Autodesk Inventor part; units mm, degrees
ref_plane "YZ Plane" through (0, 0, 0) normal (1, 0, 0) x (0, 1, 0)
ref_plane "XZ Plane" through (0, 0, 0) normal (0, 1, 0) x (-1, 0, 0)
ref_plane "XY Plane" through (0, 0, 0) normal (0, 0, 1) x (1, 0, 0)
sketch "Sketch1" plane through (0, 0, 0) normal (0, 0, 1) x (1, 0, 0)
  line L0 (-266.7, 101.6) -> (-342.9, 101.6)
  line L1 (-342.9, 101.6) -> (-342.9, 0)
  line L2 (-342.9, 0) -> (342.9, 0)
  line L3 (342.9, 0) -> (342.9, 101.6)
  line L4 (342.9, 101.6) -> (266.7, 101.6)
  line L5 (266.7, 101.6) -> (266.7, 2.54)
  line L6 (266.7, 2.54) -> (-266.7, 2.54)
  line L7 (-266.7, 2.54) -> (-266.7, 101.6)
  point P0 (0, 0)
  point P1 (0, 0)
  point P2 (0, 2.54)
  dimension "d0" = 685.8
  dimension "d1" = 101.6
  dimension "d2" = 76.2
  dimension "d3" = 2.54
extrude "Extrusion1" add sketch "Sketch1" along normal mid plane 939.8
sketch "Sketch2" plane through (0, 0, -469.9) normal (0, 0, -1) x (-1, 0, 0)
  line L0 (-342.9, 0) -> (-342.9, 101.6)
  line L1 (342.9, 0) -> (-342.9, 0)
  line L2 (-342.9, 101.6) -> (342.9, 101.6)
  line L3 (342.9, 101.6) -> (342.9, 0)
  line L4 (342.9, 0) -> (-342.9, 0)
  line L5 (-342.9, 0) -> (-342.9, 101.6)
  point P0 (0, 0)
extrude "Extrusion2" add sketch "Sketch2" along normal blind 2.54
sketch "Sketch3" plane through (-266.7, 2.54, 469.9) normal (0, 1, 0) x (1, 0, 0)
  line L0 (0, 0) -> (533.4, 0)
  line L1 (533.4, 939.8) -> (533.4, 0)
  line L2 (0, 939.8) -> (0, 0)
  line L3 (0, 152.4) -> (533.4, 152.4)
  line L4 (533.4, 152.4) -> (533.4, 228.6)
  line L5 (533.4, 228.6) -> (0, 228.6)
  line L6 (0, 228.6) -> (0, 152.4)
  line L7 (0, 533.4) -> (152.4, 533.4)
  line L8 (152.4, 533.4) -> (152.4, 406.4)
  line L9 (152.4, 406.4) -> (0, 406.4)
  line L10 (0, 406.4) -> (0, 533.4)
  line L11 (381, 533.4) -> (533.4, 533.4)
  line L12 (533.4, 533.4) -> (533.4, 406.4)
  line L13 (533.4, 406.4) -> (381, 406.4)
  line L14 (381, 406.4) -> (381, 533.4)
  point P0 (266.7, 469.9)
  point P1 (152.4, 469.9)
  dimension "d8" = 76.2
  dimension "d9" = 152.4
  dimension "d31" = 152.4
  dimension "d32" = 127
extrude "Extrusion7" cut sketch "Sketch3" against normal up to next contours L2 L3 L1 L0
extrude "Extrusion3" add sketch "Sketch3" along normal blind 25.4 contours L2 L5 L1 L3
extrude "Extrusion8" add sketch "Sketch3" along normal blind 127 contours L2 L7 L8 L9 | L13 L14 L11 L1
sketch "Sketch4" plane through (-342.9, 0, 469.9) normal (0, -1, 0) x (1, 0, 0)
  line L0 (685.8, 0) -> (0, 0)
  line L1 (0, -942.34) -> (0, 0)
  line L2 (0, -942.34) -> (685.8, -942.34)
  line L3 (76.2, -939.8) -> (76.2, -228.6)
  line L4 (342.9, -469.9) -> (342.9, 0) construction
  line L5 (12.7, -929.64) -> (63.5, -929.64)
  line L6 (63.5, -929.64) -> (63.5, -12.7)
  line L7 (63.5, -12.7) -> (12.7, -12.7)
  line L8 (12.7, -12.7) -> (12.7, -929.64)
  line L9 (673.1, -929.64) -> (622.3, -929.64)
  line L10 (622.3, -929.64) -> (622.3, -12.7)
  line L11 (622.3, -12.7) -> (673.1, -12.7)
  line L12 (673.1, -12.7) -> (673.1, -929.64)
  dimension "d12" = 12.7
  dimension "d13" = 12.7
  dimension "d14" = 12.7
  dimension "d15" = 12.7
extrude "Extrusion4" cut sketch "Sketch4" against normal blind 88.9
sketch "Sketch5" plane through (-266.7, 2.54, -469.9) normal (0, 1, 0) x (1, 0, 0)
  line L0 (533.4, 0) -> (0, 0)
  line L1 (0, 0) -> (0, -711.2)
  line L2 (152.4, -101.6) -> (165.1, -101.6)
  line L3 (165.1, -101.6) -> (165.1, -228.6)
  line L4 (165.1, -228.6) -> (152.4, -228.6)
  line L5 (152.4, -228.6) -> (152.4, -101.6)
  line L6 (228.6, -101.6) -> (241.3, -101.6)
  line L7 (241.3, -101.6) -> (241.3, -228.6)
  line L8 (241.3, -228.6) -> (228.6, -228.6)
  line L9 (228.6, -228.6) -> (228.6, -101.6)
  point P0 (266.7, -469.9)
  dimension "d18" = 12.7
  dimension "d19" = 127
  dimension "d20" = 63.5
  dimension "d21" = 152.4
  dimension "d22" = 101.6
extrude "Extrusion5" add sketch "Sketch5" along normal blind 139.7
sketch "Sketch6" plane through (-25.4, 2.54, -241.3) normal (1, 0, 0) x (0, 0, -1)
  line L0 (127, 139.7) -> (0, 139.7)
  circle A0 centre (63.5, 101.6) radius 14.2875
  point P0 (-241.3, -2.54)
  point P1 (63.5, 139.7)
  dimension "d25" = 28.575
  dimension "d26" = 38.1
extrude "Extrusion6" cut sketch "Sketch6" against normal up to surface (88.9 mm away)
properties part number "Concept"
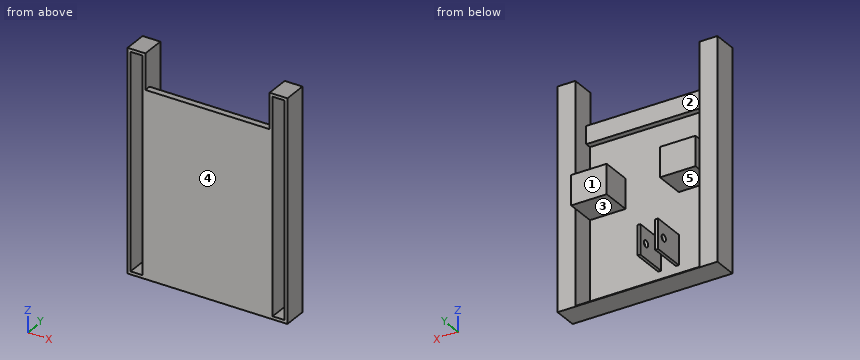
The listing builds one solid part. Answer for the finished solid, in the listing's coordinates (mm). Face numbers are marked on the shaded views. A direction names the side the tool comes from. Coordinates: 2 decimals unless noted, no trailing zeros. Write each loop counter-clockwise with the first axis right and the second up, starting at its lowest first coordinate (ties: lowest second). Pieces come first, ordered by that corner, then holes. Notation, with made-up numbers: (51, 33) - (110, 33) arc R26 ccw to (110, 70) - close; hole circle Ø9 at (0, 10). An arc over 180 degrees is marked (long way). Return JSON: item names as keys, results as strings. Group by question number.
1. Straight lines are drawn through the part: L1, parallel to X at y = 38.5, z = 87.5; L2, parallel to X at y = 71, z = -339.5; L3, parallel to X at y = 45.5, z = 0.5. For each, find the intervals that lie inside material, in ascending order.
2. A cutting plane is placed at A-A, the plane y = 77. Give the number of separate pieces and of enclosed holes in the cut face, plus the area to 3 significant figures.
3. Determine the mould class of the marked faces 4 and 5 for opening direction Z: released by +Z, released by -Z, zero draft, split by the parting line, or undercut.
4. A cutting plane is placed at C-C, the plane z = 389. Determine the outline of the cut face in (x, y).
5. A cutting plane is placed at D-D, the plane x = 32.5. Determine the outline of the cut face in (y, z).
6. Which of the six approach directions +Z, -Z, +X, -X, +Y, -Y give full straight-line access (tool end or side, diameter ignored) to the marked faces 1, 2 and 3?
7. Given pin 1 (10 mm diameter, centred on x = -34, y = 57, fed in from +Z); pin 2 (1 mm diameter, centred on x = -246, z = 295.5, fed in from +Y), each flat-ended and moving along its own axis, determine where each tip first touches the part or whether it passes through.
Ans:
{
 "1": {"L1": "-342.9 to -330.2, -279.4 to -266.7, 266.7 to 279.4, 330.2 to 342.9", "L2": "-342.9 to -330.2, -279.4 to -266.7, -114.3 to -101.6, -38.1 to -25.4, 266.7 to 279.4, 330.2 to 342.9", "L3": "-342.9 to -330.2, -279.4 to -114.3, 114.3 to 279.4, 330.2 to 342.9"},
 "2": {"separate pieces": "3", "enclosed holes": "2", "area": "93,700 mm²"},
 "3": {"face 4": "zero draft", "face 5": "undercut"},
 "4": {"outline": "(-342.9, 0) - (-330.2, 0) - (-330.2, 88.9) - (-279.4, 88.9) - (-279.4, 0) - (-266.7, 0) - (-266.7, 101.6) - (-342.9, 101.6) - close; (266.7, 0) - (279.4, 0) - (279.4, 88.9) - (330.2, 88.9) - (330.2, 0) - (342.9, 0) - (342.9, 101.6) - (266.7, 101.6) - close"},
 "5": {"outline": "(0, -472.44) - (101.6, -472.44) - (101.6, -469.9) - (2.54, -469.9) - (2.54, 241.3) - (27.94, 241.3) - (27.94, 317.5) - (0, 317.5) - close"},
 "6": {"face 1": "+Z, -Z, +X, -X, +Y", "face 2": "+Z, +Y", "face 3": "+Y"},
 "7": {"pin 1": "z = -241.3", "pin 2": "y = 27.94"}
}
